Job drawing, mm, ordinate dimensions from the low corner. One solid piece. Round coordinates to 2 decimals unless told otherwise and drop trailing zeros. Loops run counter-clockwise (first coordinate to the right, second up) from the corner with the lowest first, then second, coordinate; pieces in that order, holes last.
1) Band-saw the part on D-D, the plane x = 7. Write the cut outline in (y, z).
2) Band-saw the part on C-C, the plane z = 1.7. Write the cut outline in (x, y).
3) Band-saw the part on A-A, the plane y = 2.75. Write the cut outline in (x, z) (3 decimals), then the cut area to 3 significant figures.
4) Probe line 1 (X direction, y = 7.5, z = 1.15); line 2 (Y direction, x = 7.75, z = 1.25); line 3 (Z direction, x = 1.25, y = 9.25). List the from-to ranges inside material, lowest first.
5) Drop a flat-ended pin along its axis: P1, Ø1, axis at x = 1.5, z = 0.5, coming from the +Y side. Give the stop position or say it passes through.
6) Band-saw the part on B-B, the plane x = 11.43. Write the cut outline in (y, z).
7) Mould opens along X. For the marked faces 1, 2, 3 and 4 say: +X half, -X half, draft (parallel to the pull), parting line (faces both ways), or undercut.
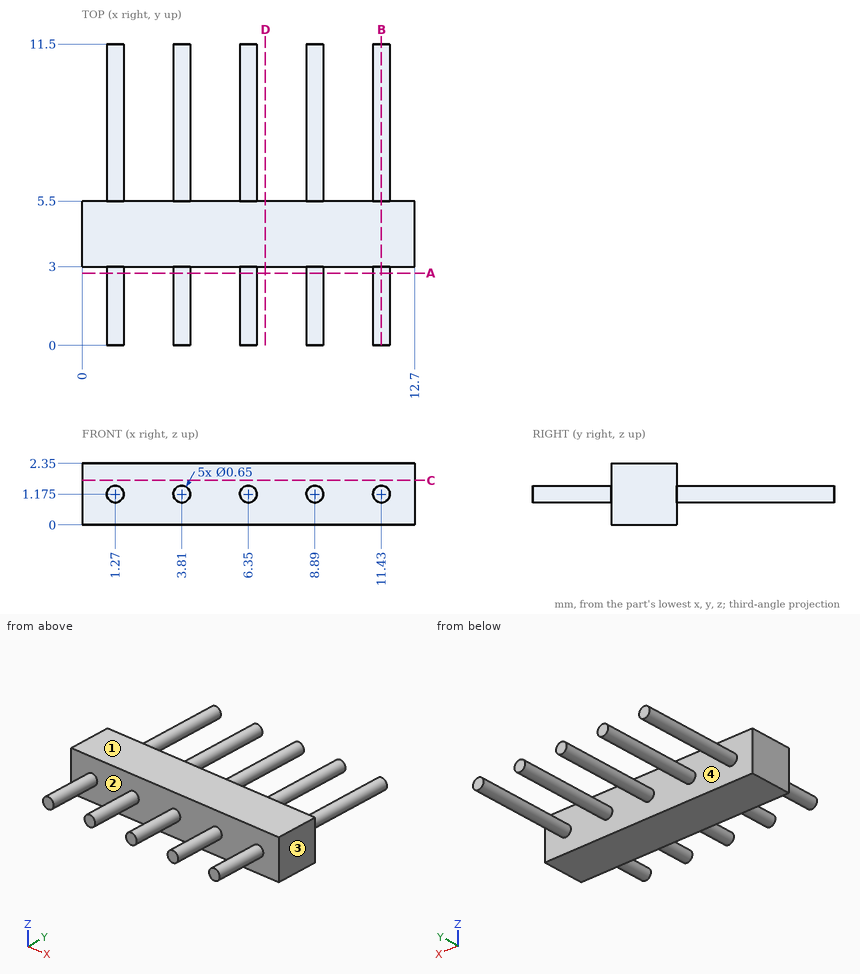
Reported:
1. outline: (3, 0) - (5.5, 0) - (5.5, 2.35) - (3, 2.35) - close
2. outline: (0, 3) - (12.7, 3) - (12.7, 5.5) - (0, 5.5) - close
3. outline: circle Ø0.65 at (1.27, 1.175); circle Ø0.65 at (3.81, 1.175); circle Ø0.65 at (6.35, 1.175); circle Ø0.65 at (8.89, 1.175); circle Ø0.65 at (11.43, 1.175)
3. area: 1.66 mm2
4. line 1: x = 0.95 to 1.59, 3.49 to 4.13, 6.03 to 6.67, 8.57 to 9.21, 11.11 to 11.75
4. line 2: y = 3 to 5.5
4. line 3: z = 0.85 to 1.5
5. P1: stops at y = 11.5
6. outline: (0, 0.85) - (3, 0.85) - (3, 0) - (5.5, 0) - (5.5, 0.85) - (11.5, 0.85) - (11.5, 1.5) - (5.5, 1.5) - (5.5, 2.35) - (3, 2.35) - (3, 1.5) - (0, 1.5) - close
7. face 1: draft
7. face 2: undercut
7. face 3: +X half
7. face 4: undercut
